```python
from build123d import *

# Parameters (mm, degrees)
EXTRUDE_1_DEPTH     = 15
FILLET_1_R          = 3
SKETCH_2_R          = 3
CUT_EXTRUDE_1_DEPTH = 32.400636936
SKETCH_3_R          = 1.5
CUT_EXTRUDE_2_DEPTH = 10
SKETCH_3_3_R        = 1.5
CUT_EXTRUDE_3_DEPTH = 10


with BuildPart() as part:
    # Sketch 1 → Extrude 1 (new body)
    with BuildSketch(Plane.XY):
        Polygon((9.5, 0), (-9.5, 0), (-9.5, 20), (-6.5, 20), (-6.5, 5), (6.5, 5), (6.5, 20), (9.5, 20), align=None)
    extrude(amount=EXTRUDE_1_DEPTH)

    # Fillet 1
    fillet_1_edges = [part.edges().sort_by_distance(p)[0] for p in [
        (-6.5, 5, 7.5),
        (6.5, 5, 7.5),
    ]]
    fillet(fillet_1_edges, radius=FILLET_1_R)

    # Sketch 2 → Cut-Extrude 1 (cut, through all)
    with BuildSketch(Plane(origin=(9.5, 0, 0), x_dir=(0, 0, -1), z_dir=(1, 0, 0))):
        with Locations(Location((-4.5, 15.5, 0), (0, 0, 90))):
            Circle(SKETCH_2_R)
    extrude(amount=-CUT_EXTRUDE_1_DEPTH, mode=Mode.SUBTRACT)

    # Sketch 3 → Cut-Extrude 2 (cut)
    with BuildSketch(Plane(origin=(0, 5, 0), x_dir=(1, 0, 0), z_dir=(0, 1, 0))):
        with Locations(Location((0, -11.5, 0), (0, 0, 270))):
            Circle(SKETCH_3_R)
    extrude(amount=-CUT_EXTRUDE_2_DEPTH, mode=Mode.SUBTRACT)

    # Sketch 3_3 → Cut-Extrude 3 (cut)
    with BuildSketch(Plane(origin=(0, 5, 0), x_dir=(1, 0, 0), z_dir=(0, 1, 0))):
        with Locations(Location((0, -11.5, 0), (0, 0, 270))):
            Circle(SKETCH_3_3_R)
        with Locations(Location((0, -3.5, 0), (0, 0, 180))):
            Circle(SKETCH_3_3_R)
    extrude(amount=-CUT_EXTRUDE_3_DEPTH, mode=Mode.SUBTRACT)


solid = part.part
```
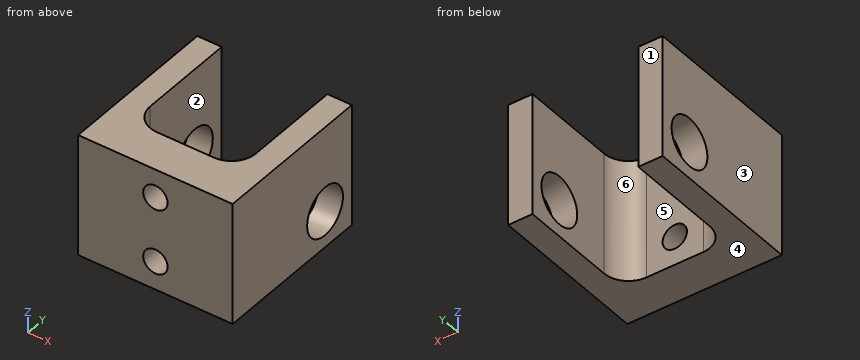
Design review of the part built by this model. Coordinates are the model's own, in mm. Face numbers are marked on the shaded views. A direction names the side the tool comes from. Give positions to 0.01 mm unless a question says otherwise; leave off trailing zeros. Write each loop counter-clockwise with the first axis right and the second up, starting at its lowest first coordinate (ties: lowest second). Pieces come first, ordered by that corner, then holes. Notation, with made-up numbers: (7, -3) - (60, -3) arc R31 ccw to (60, 31) - close; hole circle Ø3 at (2.5, -13). An arc over 180 degrees is marked (long way). Return JSON: item names as keys, results as strings. Group by question number.
(1) To check wall thickness, follow probe 1 along X at (y, z) = (15.75, 13); probe 2 along X at (y, z) = (3.5, 11.5); probe 3 along Y at (x, z) = (2, 3.75). State the ranges of each line that lie inside material, in increasing order.
(2) We need section D-D, the plane z = 4.5. Give the boundary of the cut face in (x, y), then the cut area to 3 significant figures.
(3) We need section C-C, the plane y = 6.75. Give the boundary of the cut face in (x, z).
(4) We need section B-B, the plane z = 11.5. Give the boundary of the cut face in (x, y).
(5) Insertion check: pin 1 (3.5 mm diameter, centred on y = 15.5, z = 4.5, fed in from -X); pin 2 (2 mm diameter, centred on x = -1, z = 6.5, fed in from +Y). Each pin has a flat end and moves straight along its axis. Give the tip position at first contact, or say it passes through.
(6) Mouldability with a two-part tool opening along X and no side actions: class the marked faces 3, 4, 5 and 6 as +X half, -X half, draft (parallel to the pull), parting line (faces both ways), or undercut.
(7) Machinability: for the marked faces 1 and 2, which of the approach directions +Z, -Z, +X, -X, +Y, -Y give a long, thin tool a straight path to every point of the face, cutting with its end or side? Answer none if there is none.
(8) We need section A-A, the plane x = 0. Give the boundary of the cut face in (y, z), then the cut area to 3 significant figures.
Reported:
{
 "1": {"probe 1": "x = -9.5 to -6.5, 6.5 to 9.5", "probe 2": "x = -9.5 to -1.5, 1.5 to 9.5", "probe 3": "y = 0 to 5"},
 "2": {"outline": "(-9.5, 0) - (-1.12, 0) - (-1.12, 5) - (-3.5, 5) arc R3 cw to (-6.5, 8) - (-6.5, 12.5) - (-9.5, 12.5) - close; (-9.5, 18.5) - (-6.5, 18.5) - (-6.5, 20) - (-9.5, 20) - close; (1.12, 0) - (9.5, 0) - (9.5, 12.5) - (6.5, 12.5) - (6.5, 8) arc R3 cw to (3.5, 5) - (1.12, 5) - close; (6.5, 18.5) - (9.5, 18.5) - (9.5, 20) - (6.5, 20) - close", "area": "142 mm2"},
 "3": {"outline": "(-9.5, 0) - (-6.23, 0) - (-6.23, 15) - (-9.5, 15) - close; (6.23, 0) - (9.5, 0) - (9.5, 15) - (6.23, 15) - close"},
 "4": {"outline": "(-9.5, 0) - (-1.5, 0) - (-1.5, 5) - (-3.5, 5) arc R3 cw to (-6.5, 8) - (-6.5, 20) - (-9.5, 20) - close; (1.5, 0) - (9.5, 0) - (9.5, 20) - (6.5, 20) - (6.5, 8) arc R3 cw to (3.5, 5) - (1.5, 5) - close"},
 "5": {"pin 1": "passes through", "pin 2": "stops at y = 5"},
 "6": {"face 3": "-X half", "face 4": "draft", "face 5": "undercut", "face 6": "undercut"},
 "7": {"face 1": "+Z, -Z, +X, -X, +Y", "face 2": "+Z, -Z, +Y"},
 "8": {"outline": "(0, 0) - (5, 0) - (5, 2) - (0, 2) - close; (0, 5) - (5, 5) - (5, 10) - (0, 10) - close; (0, 13) - (5, 13) - (5, 15) - (0, 15) - close", "area": "45.0 mm2"}
}
